```python
from build123d import *

# Parameters (mm, degrees)
BOSS_EXTRUDE2_DEPTH = 30
SKETCH2_W           = 2
SKETCH2_H           = 77.78174593
BOSS_EXTRUDE3_DEPTH = 10
SKETCH3_W           = 27.5
SKETCH3_H           = 30
BOSS_EXTRUDE4_DEPTH = 110
SKETCH4_R           = 12.012972295
SKETCH4_R_2         = 12
BOSS_EXTRUDE8_DEPTH = 10


with BuildPart() as part:
    # Sketch1 → Boss-Extrude2 (new body)
    with BuildSketch(Plane.XY):
        Polygon((0, 0), (0, 55), (55, 0), align=None)
    extrude(amount=-BOSS_EXTRUDE2_DEPTH)

    # Sketch2 → Boss-Extrude3 (add)
    with BuildSketch(Plane(origin=(27.5, 27.5, 0), x_dir=(0, 0, -1), z_dir=(0.7071067811865477, 0.7071067811865475, 0))):
        with Locations((1, 0)):
            Rectangle(SKETCH2_W, SKETCH2_H)
        with Locations((29, 0)):
            Rectangle(SKETCH2_W, SKETCH2_H)
    extrude(amount=BOSS_EXTRUDE3_DEPTH)

    # Sketch3 → Boss-Extrude4 (add)
    with BuildSketch(Plane.XZ):
        with Locations((13.75, -15)):
            Rectangle(SKETCH3_W, SKETCH3_H)
    extrude(amount=BOSS_EXTRUDE4_DEPTH)

    # Sketch4 → Boss-Extrude8 (add)
    with BuildSketch(Plane(origin=(27.5, 27.5, 0), x_dir=(0, 0, -1), z_dir=(0.7071067811865477, 0.7071067811865475, 0))):
        with Locations(Location((15, -26.87790067, 0), (0, 0, 270))):
            Circle(SKETCH4_R)
        with Locations(Location((15, -2.860782845, 0), (0, 0, 90))):
            Circle(SKETCH4_R_2)
        with Locations(Location((15, 21.143362684, 0), (0, 0, 90))):
            Circle(SKETCH4_R_2)
    extrude(amount=BOSS_EXTRUDE8_DEPTH)


solid = part.part
```
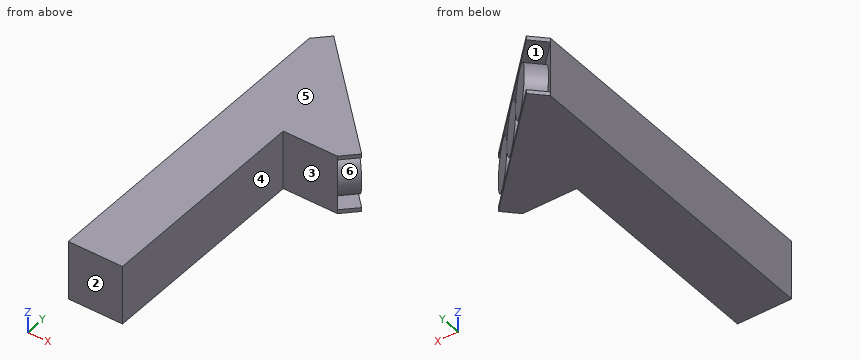
Work out the finished part from the listing and answer in its coordinate system (mm). Face numbers are marked on the shaded views. A direction names the side the tool comes from. Round coordinates to 2 decimals unless told otherwise and drop trailing zeros. Loops run counter-clockwise (first coordinate to the right, second up) from the corner with the lowest first, then second, coordinate; pieces in that order, holes last.
(1) Find the intervals of material crossed by L1, parallel to X at y = -13, z = -19.5; L2, parallel to X at y = 18.5, z = -24.75; L3, parallel to Y at x = 23.5, z = -13, in increasing order.
Computed values:
L1: x = 0 to 27.5
L2: x = 0 to 36.5, 46.59 to 50.64
L3: y = -110 to 36.19, 36.67 to 45.64
(2) For the marked faces 1, 2 and 3, determine the directions among +Z, -Z, +X, -X, +Y, -Y from which every point of the face is accessible in a straight line to the end or side of a thin tool.
Computed values:
face 1: +X, +Y
face 2: +Z, -Z, +X, -X, -Y
face 3: +Z, -Z, +X, -Y
(3) The part is cut by section C-C, the plane x = 57.5. Give the number of separate pieces and of enclosed holes in the cut face, and give its area (3 significant figures).
Computed values:
separate pieces: 3
enclosed holes: 0
area: 176 mm2
(4) The mould has two halves that part along X. Classify the marked faces 4, 5 and 6: pulls with the +X half, pulls with the -X half, needs draft (parallel to the pull), parting line crosses it, or undercut.
Computed values:
face 4: pulls with the +X half
face 5: needs draft
face 6: undercut
(5) The part is cut by section A-A, the plane z = -6.75. Give the vertices of the cut face in (x, y), and give its area (3 significant figures).
Computed values:
outline: (0, -110) - (27.5, -110) - (27.5, 0) - (55, 0) - (52.68, 2.32) - (59.75, 9.39) - (47.4, 21.74) - (40.33, 14.67) - (35.68, 19.32) - (42.76, 26.39) - (30.43, 38.71) - (23.36, 31.64) - (18.71, 36.29) - (25.78, 43.36) - (13.46, 55.68) - (6.39, 48.61) - (0, 55) - close
area: 5,060 mm2
(6) The part is cut by section B-B, the plane y = -23.5. Give the vertices of the cut face in (x, z), and give its area (3 significant figures).
Computed values:
outline: (0, -30) - (27.5, -30) - (27.5, 0) - (0, 0) - close
area: 825 mm2
(7) Each of these flat-tipped pins is pushed along its axis until it touches: P1, Ø8, axis at x = 43, z = -11.5, coming from the -Y side; P2, Ø1.5, axis at x = 31, z = -24, coming from the +Y side; P3, Ø1.5, axis at y = -43.5, z = -12, coming from the +X side. Where does it stop, or does it pass through?
Computed values:
P1: stops at y = 0
P2: stops at y = 38.6
P3: stops at x = 27.5
(8) The part is cut by section D-D, the plane z = -18.5. Give the vertices of the cut face in (x, y), and give its area (3 significant figures).
Computed values:
outline: (0, -110) - (27.5, -110) - (27.5, 0) - (55, 0) - (54.63, 0.37) - (61.7, 7.44) - (45.45, 23.69) - (38.38, 16.62) - (37.64, 17.36) - (44.71, 24.43) - (28.48, 40.66) - (21.41, 33.59) - (20.67, 34.33) - (27.74, 41.41) - (11.5, 57.64) - (4.43, 50.57) - (0, 55) - close
area: 5,230 mm2
